from build123d import *

# Parameters (mm, degrees)
SZKIC1_R                    = 1.95
DODANIE_WYCI_GNI_CIE1_DEPTH = 165
SZKIC2_R                    = 8.5
DODANIE_WYCI_GNI_CIE2_DEPTH = 3
SZKIC6_R                    = 0.75
WYTNIJ_WYCI_GNI_CIE2_DEPTH  = 11


with BuildPart() as part:
    # Szkic1 → Dodanie-wyciągnięcie1 (new body)
    with BuildSketch(Plane.XY):
        Circle(SZKIC1_R)
    extrude(amount=DODANIE_WYCI_GNI_CIE1_DEPTH)

    # Szkic2 → Dodanie-wyciągnięcie2 (add)
    with BuildSketch(Plane.XY.offset(165)):
        Circle(SZKIC2_R)
    extrude(amount=DODANIE_WYCI_GNI_CIE2_DEPTH)

    # Szkic6 → Wytnij-wyciągnięcie2 (cut)
    with BuildSketch(Plane.ZY.offset(1.95)):
        with Locations((15, 0)):
            Circle(SZKIC6_R)
    extrude(amount=-WYTNIJ_WYCI_GNI_CIE2_DEPTH, mode=Mode.SUBTRACT)


solid = part.part
Geometry: final body of the model. Coordinates: model frame, mm. A direction names the side the tool comes from. Round coordinates to 2 decimals unless told otherwise and drop trailing zeros. Loops run counter-clockwise (first coordinate to the right, second up) from the corner with the lowest first, then second, coordinate; pieces in that order, holes last.
Q1. Pin query (flat end, axial travel): P1, Ø5, axis at x = -1, z = 43, coming from the +Y side; P2, Ø2, axis at x = 3.5, z = 45, coming from the -Y side; P3, Ø10, axis at y = 2, z = 98.5, coming from the +X side; P4, Ø8, axis at x = -2, z = 59.5, coming from the -Y side. Return the tip coordinate at first contact, or that it passes through.
Q2. Access query for faces 1 (the cylindrical face through (-1.437, 1.318, 81.345)), 2 (the cylindrical face through (4.57, 7.167, 166.479)). Directions: +Z, -Z, +X, -X, +Y, -Y. A direction counts if a zero-diameter tool reaches every point of the face in a straight line with its end or side. Return the directions, or none.
Q3. Section D-D on x = 6.5. Return loops of the section in (y, z), plus the area to 3 significant figures.
Q4. Section A-A on x = 0. Return loops of the section in (y, z), plus the area to 3 significant figures.
Q5. Section B-B on y = 4. Return loops of the section in (x, z).
Q6. Material intervals for L1, parallel to Z at x = 0.5, y = 0; L2, parallel to Z at x = -5.75, y = -0.75; L3, parallel to Y at x = 1, z = 15, sorted ascending.
Q7. Section C-C on z = 127. Return loops of the section in (x, y), plus the area to 3 significant figures.
Evaluation:
1. P1: stops at y = 1.95
1. P2: passes through
1. P3: stops at x = 1.95
1. P4: stops at y = -1.95
2. face 1: -Z
2. face 2: +Z, -Z
3. outline: (-5.48, 165) - (5.48, 165) - (5.48, 168) - (-5.48, 168) - close
3. area: 32.9 mm2
4. outline: (-8.5, 165) - (-1.95, 165) - (-1.95, 0) - (1.95, 0) - (1.95, 165) - (8.5, 165) - (8.5, 168) - (-8.5, 168) - close; hole circle Ø1.5 at (0, 15)
4. area: 693 mm2
5. outline: (-7.5, 165) - (7.5, 165) - (7.5, 168) - (-7.5, 168) - close
6. L1: z = 0 to 14.25, 15.75 to 168
6. L2: z = 165 to 168
6. L3: y = -1.67 to -0.75, 0.75 to 1.67
7. outline: circle Ø3.9 at (0, 0)
7. area: 11.9 mm2
